```python
from build123d import *

# Parameters (mm, degrees)
F0_W      = 50.8
F0_H      = 50.8
F1_DEPTH  = 3.81
F2_W      = 50.8
F2_H      = 2.54
F3_DEPTH  = 12.7
F4_W      = 20.955
F4_H      = 2.54
F5_DEPTH  = 12.7
F6_W      = 20.955
F6_H      = 2.54
F7_DEPTH  = 2.54
F8_W      = 3.81
F8_H      = 45.72
F9_DEPTH  = 2.54
F10_DEPTH = 10.16
F11_W     = 6.35
F11_H     = 8.89
F12_DEPTH = 25.4
F13_W     = 6.35
F13_H     = 8.89
F14_DEPTH = 25.4


with BuildPart() as f1:
    # F0 (on Top) → F1 (new body)
    with BuildSketch(Plane.XY):
        with Locations((-6.6145006567, 7.1719978217)):
            Rectangle(F0_W, F0_H)
    extrude(amount=F1_DEPTH)

    # F2 (on face) → F3 (join)
    with BuildSketch(Plane.XY.offset(3.81)):
        with Locations((-6.6145006567, 31.3019978217)):
            Rectangle(F2_W, F2_H)
    extrude(amount=F3_DEPTH)

    # F4 (on face) → F5 (join)
    with BuildSketch(Plane.XY.offset(3.81)):
        with Locations((-21.5370006567, -16.9580021783)):
            Rectangle(F4_W, F4_H)
    extrude(amount=F5_DEPTH)

    # F6 (on face) → F7 (join)
    with BuildSketch(Plane.XY.offset(3.81)):
        with Locations((8.3079993433, -16.9580021783)):
            Rectangle(F6_W, F6_H)
    extrude(amount=F7_DEPTH)

    # F8 (on face) → F9 (join)
    with BuildSketch(Plane.XY.offset(3.81)):
        with Locations((16.8804993433, 7.1719978217)):
            Rectangle(F8_W, F8_H)
    extrude(amount=F9_DEPTH)

    # F10 (add): a face of the model
    f10_faces = [f1.faces().sort_by_distance(p)[0] for p in [
        (6.4029993433, -16.214133305, 6.35),
    ]]
    extrude(f10_faces, amount=F10_DEPTH)

    # F11 (on face) → F12 (join)
    with BuildSketch(Plane.XY.offset(3.81)):
        with Locations((-2.8045006567, -7.122488919)):
            Rectangle(F11_W, F11_H)
    extrude(amount=F12_DEPTH)

    # F13 (on face) → F14 (join)
    with BuildSketch(Plane.XY.offset(3.81)):
        with Locations((-2.8045006567, 23.80011379)):
            Rectangle(F13_W, F13_H)
    extrude(amount=F14_DEPTH)


solid = f1.part
```
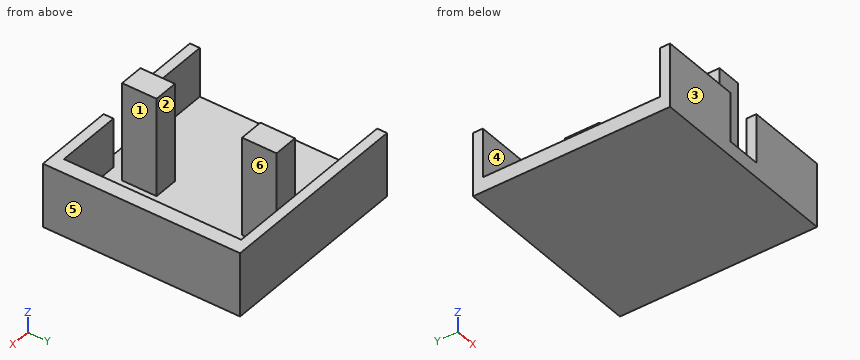
Source: CAD feature listing. Evaluate the final solid. Frame: model axes, mm. Face numbers are marked on the shaded views. A direction names the side the tool comes from. Coordinates: 2 decimals unless noted, no trailing zeros. Loops run counter-clockwise (first coordinate to the right, second up) from the corner with the lowest first, then second, coordinate; pieces in that order, holes last. Notation, with made-up numbers: M 72,0.5 L 103,0.5 A21 cw 103,39.5 Z; hole C 42.25,49 d6. An arc over 180 degrees is marked long. Use a Markdown table: item, result. Add a question column.
Q1. Section query A-A, the plane z = 8.5. Return loops of the section in (x, y), and give its area (3 significant figures).
Q2. Material intervals for L1, parallel to Y at x = 1, z = 9.5; L2, parallel to X at y = -11, z = 7.75; L3, parallel to Z at x = -13, y = 12, sorted ascending.
Q3. Section query D-D, the plane y = 17.5. Return loops of the section in (x, z).
Q4. Section query C-C, the plane x = -1.5. Return loops of the section in (y, z), and give its area (3 significant figures).
Q5. Draft query along X for the marked faces 4, 5 and 6. Return one class per face: pulls with the +X half, pulls with the -X half, needs draft (parallel to the pull), parting line crosses it, or undercut.
Q6. Section query B-B, the plane z = 26.25. Return loops of the section in (x, y), and give its area (3 significant figures).
Q7. Access query for the marked faces 1, 2 and 3. Directions: +Z, -Z, +X, -X, +Y, -Y. A direction counts if a zero-diameter tool reaches every point of the face in a straight line with its end or side. Return the directions, or none.
Q8. First-contact query: pin 1 (5 mm diameter, centred on x = -2.5, z = 21, fed in from -Y); pin 2 (3 mm diameter, centred on x = -20, y = -17.5, fed in from +Z); pin 3 (4.5 mm diameter, centred on y = 24, z = 15.5, fed in from -X). Flat tips, straight axial feed; report the tip coordinate or a pass-through.
Result:
| question | item | result |
|---|---|---|
| 1 | outline | M -32.01,-18.23 L -11.06,-18.23 L -11.06,-15.69 L -32.01,-15.69 Z; M -32.01,30.03 L 14.98,30.03 L 14.98,-15.69 L -2.17,-15.69 L -2.17,-18.23 L 18.79,-18.23 L 18.79,32.57 L -32.01,32.57 Z; M -5.98,-11.57 L 0.37,-11.57 L 0.37,-2.68 L -5.98,-2.68 Z; M -5.98,19.36 L 0.37,19.36 L 0.37,28.25 L -5.98,28.25 Z |
| 1 | area | 523 mm2 |
| 2 | L1 | y = -18.23 to -15.69, 30.03 to 32.57 |
| 2 | L2 | x = -5.98 to 0.37, 14.98 to 18.79 |
| 2 | L3 | z = 0 to 3.81 |
| 3 | outline | M -32.01,0 L 18.79,0 L 18.79,16.51 L 14.98,16.51 L 14.98,3.81 L -32.01,3.81 Z |
| 4 | outline | M -18.23,0 L 32.57,0 L 32.57,16.51 L 30.03,16.51 L 30.03,3.81 L 28.25,3.81 L 28.25,29.21 L 19.36,29.21 L 19.36,3.81 L -2.68,3.81 L -2.68,29.21 L -11.57,29.21 L -11.57,3.81 L -15.69,3.81 L -15.69,16.51 L -18.23,16.51 Z |
| 4 | area | 710 mm2 |
| 5 | face 4 | needs draft |
| 5 | face 5 | pulls with the +X half |
| 5 | face 6 | undercut |
| 6 | outline | M -5.98,-11.57 L 0.37,-11.57 L 0.37,-2.68 L -5.98,-2.68 Z; M -5.98,19.36 L 0.37,19.36 L 0.37,28.25 L -5.98,28.25 Z |
| 6 | area | 113 mm2 |
| 7 | face 1 | +Z |
| 7 | face 2 | +Z, -X |
| 7 | face 3 | +Z, -Z, +X, -X, -Y |
| 8 | pin 1 | stops at y = -11.57 |
| 8 | pin 2 | stops at z = 16.51 |
| 8 | pin 3 | stops at x = -5.98 |
